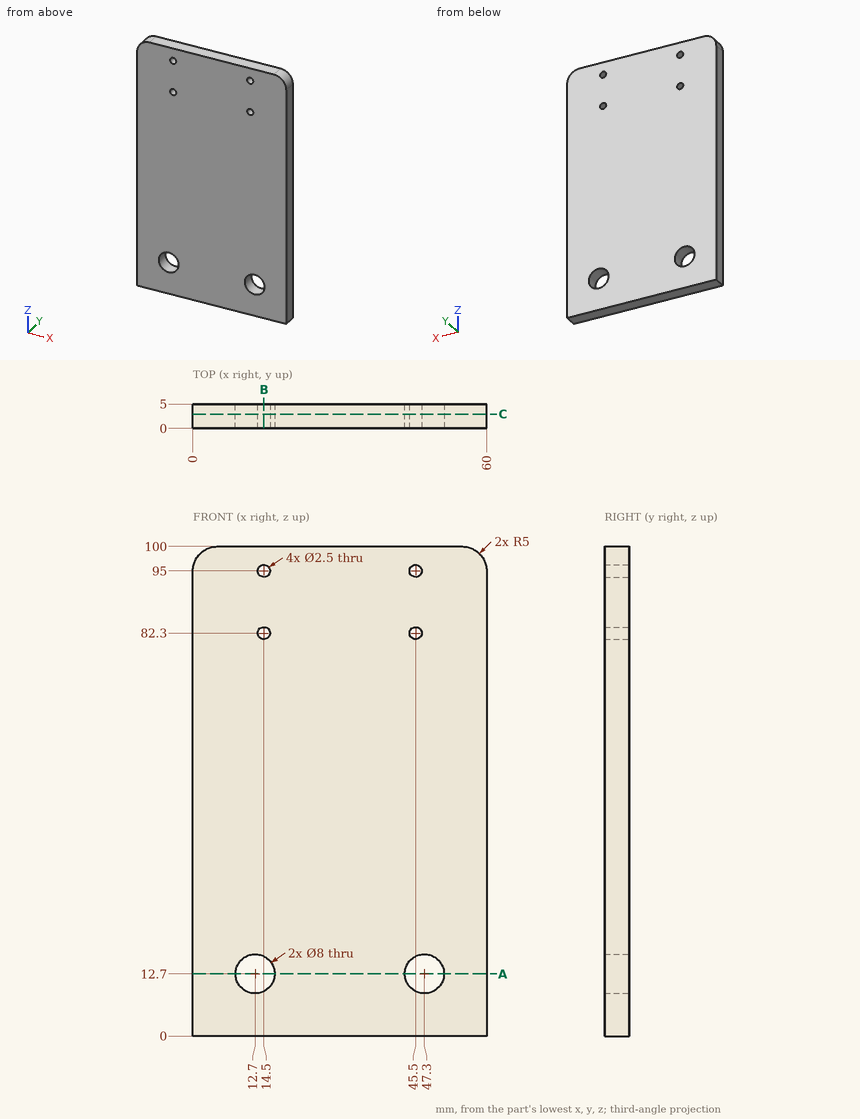
Source: three-view drawing plus pictorial views. Frame: mm from the lowest corner of the part. Round coordinates to 2 decimals unless told otherwise and drop trailing zeros. Order: outer loops, then holes, each group sorted by start corner. A loop starts at its lowest first (then second) coordinate and runs counter-clockwise, first axis right, second up. Notation, with made-up numbers: (67, -6) -> (85, -6) arc R9 ccw to (85, 0) -> close; hole circle Ø4 at (82.25, 78.5). An arc over 180 degrees is marked (long way). Use one line per item in the form item = value. Start each with the question number.
1. Cut plane A-A (z = 12.7). Return the cut outline in (x, y), then the cut area to 3 significant figures.
2. Pin query (flat end, axial travel): pin 1 Ø3 at (y, z) = (4, 58) entering from -X. Return the tip coordinate at first contact, or that it passes through.
3. Cut plane C-C (y = 2.95). Return the cut outline in (x, z), then the cut area to 3 significant figures.
4. Cut plane B-B (x = 14.5). Return the cut outline in (y, z).
5. Line query: probe 1 along X at (y, z) = (1.75, 95); probe 2 along Z at (x, y) = (14.5, 1.4); probe 3 along Z at (x, y) = (13.5, 3.4). Output: solid intervals per line, ascending.
Solution:
q1.outline = (0, 0) -> (8.7, 0) -> (8.7, 5) -> (0, 5) -> close; (16.7, 0) -> (43.3, 0) -> (43.3, 5) -> (16.7, 5) -> close; (51.3, 0) -> (60, 0) -> (60, 5) -> (51.3, 5) -> close
q1.area = 220 mm^2
q2.pin_1 = 0
q3.outline = (0, 0) -> (60, 0) -> (60, 95) arc R5 ccw to (55, 100) -> (5, 100) arc R5 ccw to (0, 95) -> close; hole circle Ø8 at (12.7, 12.7); hole circle Ø2.5 at (14.5, 82.3); hole circle Ø2.5 at (14.5, 95); hole circle Ø8 at (47.3, 12.7); hole circle Ø2.5 at (45.5, 82.3); hole circle Ø2.5 at (45.5, 95)
q3.area = 5,870 mm^2
q4.outline = (0, 0) -> (5, 0) -> (5, 9.13) -> (0, 9.13) -> close; (0, 16.27) -> (5, 16.27) -> (5, 81.05) -> (0, 81.05) -> close; (0, 83.55) -> (5, 83.55) -> (5, 93.75) -> (0, 93.75) -> close; (0, 96.25) -> (5, 96.25) -> (5, 100) -> (0, 100) -> close
q5.probe_1 = 0 to 13.25, 15.75 to 44.25, 46.75 to 60
q5.probe_2 = 0 to 9.13, 16.27 to 81.05, 83.55 to 93.75, 96.25 to 100
q5.probe_3 = 0 to 8.78, 16.62 to 81.55, 83.05 to 94.25, 95.75 to 100
